Autodesk Inventor part; units mm, degrees
ref_plane "YZ Plane" through (0, 0, 0) normal (1, 0, 0) x (0, 1, 0)
ref_plane "XZ Plane" through (0, 0, 0) normal (0, 1, 0) x (-1, 0, 0)
ref_plane "XY Plane" through (0, 0, 0) normal (0, 0, 1) x (1, 0, 0)
sketch "Sketch1" plane through (0, 0, 0) normal (0, 0, 1) x (1, 0, 0)
  line L0 (-45, 55) -> (45, 55)
  line L1 (45, 55) -> (45, -55)
  line L2 (45, -55) -> (-45, -55)
  line L3 (-45, -55) -> (-45, 55)
  point P0 (0, 0)
  point P1 (0, 55)
  point P2 (-45, 0)
  dimension "d0" = 110
  dimension "d1" = 90
extrude "Extrusion1" add sketch "Sketch1" along normal mid plane 85
sketch "Sketch2" plane through (0, 0, 42.5) normal (0, 0, 1) x (1, 0, 0)
  line L0 (-40, 50) -> (40, 50)
  line L1 (40, 50) -> (40, -50)
  line L2 (40, -50) -> (-40, -50)
  line L3 (-40, -50) -> (-40, 50)
  line L4 (45, 55) -> (-45, 55)
  line L5 (-45, 55) -> (-45, -55)
  point P0 (0, 0)
  point P1 (0, 50)
  point P2 (0, -50)
  point P3 (-40, 0)
  point P4 (40, 0)
  dimension "d6" = 5
  dimension "d7" = 5
extrude "Extrusion2" cut sketch "Sketch2" against normal blind 80
sketch "Sketch3" plane through (-45, 55, 42.5) normal (0, 1, 0) x (1, 0, 0)
  line L0 (2, 7) -> (88, 7)
  line L1 (88, 7) -> (88, 2)
  line L2 (2, 2) -> (2, 7)
  line L3 (90, 0) -> (0, 0)
  line L4 (0, 85) -> (0, 0)
  line L5 (7, 2) -> (7, 0)
  line L6 (85, 0) -> (5, 0)
  line L7 (83, 2) -> (83, 0)
  line L8 (88, 2) -> (83, 2)
  line L9 (7, 2) -> (2, 2)
  line L10 (7, 0) -> (83, 0)
  point P0 (45, 42.5)
  point P1 (45, 7)
  point P2 (2, 4.5)
  point P3 (7, 0)
  dimension "d14" = 2
  dimension "d15" = 5
  dimension "d16" = 7
  dimension "d17" = 7
  dimension "d18" = 7
  dimension "d19" = 5
extrude "Extrusion3" cut sketch "Sketch3" against normal up to surface (105 mm away)
sketch "Sketch4" plane through (-40, -50, 42.5) normal (0, 1, 0) x (1, 0, 0)
  line L0 (-3, 7) -> (83, 7)
  line L1 (83, 7) -> (83, 2)
  line L2 (83, 2) -> (-3, 2)
  line L3 (-3, 2) -> (-3, 7)
  line L4 (80, 0) -> (0, 0)
  point P0 (40, 42.5)
  point P1 (40, 2)
  point P2 (40, 0)
  point P3 (83, 4.5)
  point P4 (-3, 4.5)
  dimension "d22" = 2
  dimension "d23" = 86
  dimension "d24" = 5
extrude "Extrusion4" cut sketch "Sketch4" against normal blind 3
sketch "Sketch5" plane through (-40, -50, -37.5) normal (0, 1, 0) x (1, 0, 0)
  line L0 (80, 0) -> (0, 0)
  line L1 (11.85, -8) -> (68.15, -8)
  line L2 (68.15, -8) -> (68.15, -62.2)
  line L3 (68.15, -62.2) -> (11.85, -62.2)
  line L4 (11.85, -62.2) -> (11.85, -8)
  point P0 (40, -37.5)
  point P1 (40, -8)
  dimension "d37" = 56.3
  dimension "d38" = 54.2
  dimension "d39" = 8
sketch "Sketch6" plane through (-40, -50, -37.5) normal (0, 1, 0) x (1, 0, 0)
  line L0 (9.85, -6) -> (70.15, -6)
  line L1 (70.15, -6) -> (70.15, -64.2)
  line L2 (70.15, -64.2) -> (9.85, -64.2)
  line L3 (9.85, -64.2) -> (9.85, -6)
  line L4 (80, 0) -> (0, 0)
  point P0 (40, -37.5)
  point P1 (40, -6)
  dimension "d40" = 58.2
  dimension "d41" = 60.3
  dimension "d42" = 6
extrude "Extrusion5" add sketch "Sketch6" along normal blind 15
extrude "Extrusion6" cut sketch "Sketch5" along normal up to surface (15 mm away)
sketch "Sketch8" plane through (-40, -50, -37.5) normal (0, 1, 0) x (1, 0, 0)
  line L0 (11.85, -8) -> (68.15, -8)
  line L1 (68.15, -8) -> (68.15, -62.2)
  line L2 (11.85, -8) -> (68.15, -8)
  line L3 (68.15, -8) -> (68.15, -13)
  line L4 (68.15, -13) -> (11.85, -13)
  line L5 (11.85, -13) -> (11.85, -8)
  point P0 (40, -37.5)
  dimension "d48" = 5
extrude "Extrusion7" add sketch "Sketch8" along normal blind 4
sketch "Sketch10" plane through (-40, -50, -37.5) normal (1, 0, 0) x (0, 0, -1)
  line L0 (-25.5, 83) -> (-36.5, 83)
  line L1 (-36.5, 83) -> (-36.5, 29.5)
  line L2 (-36.5, 29.5) -> (-25.5, 29.5)
  line L3 (-25.5, 29.5) -> (-25.5, 83)
  line L4 (-8, 4) -> (-8, 15)
  line L5 (0, 0) -> (0, 100)
  line L6 (-13, 0) -> (-62.2, 0)
  point P0 (-37.5, 50)
  dimension "d52" = 25.5
  dimension "d53" = 11
  dimension "d54" = 29.5
  dimension "d55" = 53.5
extrude "Extrusion8" cut sketch "Sketch10" against normal up to surface (5 mm away)
sketch "Sketch11" plane through (-40, -50, -37.5) normal (1, 0, 0) x (0, 0, -1)
  line L0 (-38, 84.5) -> (-24, 84.5)
  line L1 (-24, 84.5) -> (-24, 28)
  line L2 (-24, 28) -> (-38, 28)
  line L3 (-38, 28) -> (-38, 84.5)
  line L4 (-36.5, 83) -> (-25.5, 83)
  line L5 (-36.5, 29.5) -> (-36.5, 83)
  point P0 (-37.5, 50)
  point P1 (-31, 84.5)
  point P2 (-31, 83)
  point P3 (-38, 56.25)
  point P4 (-36.5, 56.25)
  dimension "d58" = 1.5
  dimension "d59" = 1.5
extrude "Extrusion9" add sketch "Sketch11" along normal up to surface (11.85 mm away)
sketch "Sketch12" plane through (-28.15, -22, 0.5) normal (1, 0, 0) x (0, 0, -1)
  line L0 (12.5, 1.5) -> (12.5, 55)
  line L1 (1.5, 55) -> (12.5, 55)
  line L2 (12.5, 55) -> (12.5, 1.5)
  line L3 (12.5, 1.5) -> (1.5, 1.5)
  line L4 (1.5, 1.5) -> (1.5, 55)
  line L5 (14, 56.5) -> (0, 56.5)
  line L6 (0, 56.5) -> (0, 0)
  point P0 (0.5, 22)
  point P1 (7, 55)
  point P2 (7, 56.5)
  point P3 (0, 28.25)
  point P4 (1.5, 28.25)
  dimension "d62" = 1.5
extrude "Extrusion10" cut sketch "Sketch12" against normal up to surface (11.85 mm away)
properties part number "Part_C1"
Could you check a few things on this model? Use its own coordinates, in mm. A direction names the side the tool comes from. Round coordinates to 2 decimals unless told otherwise and drop trailing zeros. Write each loop counter-clockwise with the first axis right and the second up, starting at its lowest first coordinate (ties: lowest second). Pieces come first, ordered by that corner, then holes. Notation, with made-up numbers: (-16, 88) - (33, 88) arc R13 ccw to (33, 95) - close; hole circle Ø2 at (37, 42.25). An arc over 180 degrees is marked (long way). Put each result on its own line as item: value. Start each with the question number.
(1) For faces 1 (the flat face through (0, -43, 24.7)), 2 (the flat face through (-43, 2, 38)), 3 (the flat face through (-40.2, -12, 42.5)), 4 (the flat face through (0, -43, 26.7)), which set-ups out of +Z, -Z, +X, -X, +Y, -Y let a thin tool reach every point of the face, with its end or its side?
(2) I want a section at A-A, the plane x = -36. Please give me the cut outline in (y, z), plus the area to 3 significant figures.
(3) I want a section at C-C, the plane z = 19.5. Please give me the cut outline in (x, y), plus the area to 3 significant figures.
(4) I want a section at B-B, the plane y = -43.5. Please give me the cut outline in (x, z), plus the area to 3 significant figures.
(5) Will these pins go through, and if not, where does the flat tip stop? pin 1 (12 mm diameter, centred on x = 15.5, y = 29.5, fed in from +Z); pin 2 (1 mm diameter, centred on x = 6.5, z = 41, fed in from +Y); pin 3 (1.5 mm diameter, centred on x = -7, z = 38.5, fed in from +Y).
(6) Thinking about a two-plate mould opening in Y: for faces 5 (the flat face through (-1, 55, -10)), 6 (the flat face through (-28.15, 8.5, -0.8)), 7 (the flat face through (45, 1, -1)), which applies, released by +Y, released by -Y, zero draft, split by the parting line, or undercut?
(7) I need wall thicknesses on probe 1 along Z at (x, y) = (-6, -43.5); probe 2 along Y at (x, z) = (22.5, 10); probe 3 along X at (y, z) = (-37, -1). Which ranges of each line are inside material? Lowest first, please.
(8) I want a section at D-D, the plane y = 2. Please give me the cut outline in (x, z), plus the area to 3 significant figures.
Here are the results:
1. face 1: none
1. face 2: +Y
1. face 3: +Z, +X, -X, +Y, -Y
1. face 4: +Z
2. outline: (-55, -42.5) - (55, -42.5) - (55, 35.5) - (50, 35.5) - (50, -37.5) - (-50, -37.5) - (-50, 35.5) - (-53, 35.5) - (-53, 40.5) - (-50, 40.5) - (-50, 42.5) - (-55, 42.5) - close; (-22, -13.5) - (34.5, -13.5) - (34.5, 0.5) - (-22, 0.5) - close; hole (-20.5, -12) - (33, -12) - (33, -1) - (-20.5, -1) - close
2. area: 1,500 mm^2
3. outline: (-45, -55) - (45, -55) - (45, 55) - (-45, 55) - close; hole (-40, -50) - (-30.15, -50) - (-30.15, -35) - (-28.15, -35) - (-28.15, -50) - (28.15, -50) - (28.15, -35) - (30.15, -35) - (30.15, -50) - (40, -50) - (40, 50) - (-40, 50) - close
3. area: 1,960 mm^2
4. outline: (-45, -42.5) - (45, -42.5) - (45, 42.5) - (40, 42.5) - (40, 40.5) - (43, 40.5) - (43, 35.5) - (40, 35.5) - (40, -37.5) - (-40, -37.5) - (-40, 35.5) - (-43, 35.5) - (-43, 40.5) - (-40, 40.5) - (-40, 42.5) - (-45, 42.5) - close; (-30.15, -31.5) - (30.15, -31.5) - (30.15, 26.7) - (-30.15, 26.7) - close; hole (-28.15, -29.5) - (28.15, -29.5) - (28.15, 24.7) - (-28.15, 24.7) - close
4. area: 1,680 mm^2
5. pin 1: stops at z = -37.5
5. pin 2: stops at y = -50
5. pin 3: stops at y = -53
6. face 5: released by +Y
6. face 6: undercut
6. face 7: zero draft
7. probe 1: z = -42.5 to -37.5, -31.5 to -29.5, 24.7 to 26.7
7. probe 2: y = -55 to -50, 50 to 55
7. probe 3: x = -45 to -40, -30.15 to -28.15, 28.15 to 30.15, 40 to 45
8. outline: (-45, -42.5) - (45, -42.5) - (45, 42.5) - (40, 42.5) - (40, 40.5) - (43, 40.5) - (43, 35.5) - (40, 35.5) - (40, -37.5) - (-40, -37.5) - (-40, -13.5) - (-28.15, -13.5) - (-28.15, -12) - (-45, -12) - close; (-45, -1) - (-28.15, -1) - (-28.15, 0.5) - (-40, 0.5) - (-40, 35.5) - (-43, 35.5) - (-43, 40.5) - (-40, 40.5) - (-40, 42.5) - (-45, 42.5) - close
8. area: 1,200 mm^2
